Can you work these out from the model? Positions are in its coordinate system, mm. Give positions to 0.01 mm unless a question says otherwise; leave off trailing zeros. Loops run counter-clockwise (first coordinate to the right, second up) from the corner with the lowest first, then second, coordinate; pieces in that order, holes last. Notation, with made-up numbers: (-4.75, 23.25) - (12.25, 23.25) arc R27 ccw to (12.25, 53.25) - close; hole circle Ø6 at (-21, 11). An arc over 180 degrees is marked (long way). Answer in a Markdown table with one row per item.
Solid Edge part; units mm, degrees
sketch "Sketch1" plane through (0, 0, 0) normal (1, 0, 0) x (0, 1, 0)
  line L0 (0, 11) -> (17.9215, 11)
  line L1 (20, 9.8) -> (17.9215, 11)
  line L2 (20, 0) -> (20, 9.8)
  line L3 (0, 0) -> (20, 0)
  line L4 (0, 0) -> (0, 11)
revolve "RevolvedProtrusion1" add sketch "Sketch1" angle 360 about axis through (0, -25, 0) along (0, 1, 0)
chamfer "Chaflán_1" distance 0.2 angle 45 1 edges at (0, 0, 11)
hole "Agujero_1" at (0, 0, 0) direction (0, 1, 0) diameter 17 end up to next
Q1. If we mould it in two halves opening along X, with no side actions, what happens to faces 1 (the face through (9, 20, 0)), 2 (the face through (-10.74, 9.18, -2.38)), 3 (the face through (7.167, 9.86, -4.57))? For each: released by +X, released by -X, zero draft, split by the parting line, or undercut.
Checked values:
| item | result |
|---|---|
| face 1 | zero draft |
| face 2 | split by the parting line |
| face 3 | undercut |
Q2. Imagine slicing it at C-C, the plane y = 11.5. Write out the boundary of the cut face in (x, z), and give its area (3 significant figures).
Checked values:
| item | result |
|---|---|
| outline | circle Ø22 at (0, 0); hole circle Ø17 at (0, 0) |
| area | 153 mm² |
Q3. Imagine slicing it at B-B, the plane z = 0. Write out the boundary of the cut face in (x, y).
Checked values:
| item | result |
|---|---|
| outline | (-11, 0.2) - (-10.8, 0) - (-8.5, 0) - (-8.5, 20) - (-9.8, 20) - (-11, 17.92) - close; (8.5, 0) - (10.8, 0) - (11, 0.2) - (11, 17.92) - (9.8, 20) - (8.5, 20) - close |
Q4. If I drill on line 1 (X direction, y = 9.75, z = 0); line 2 (X direction, y = 7.5, z = -4), over which ranges is the centre line in solid material (lowest first)? Write a range as [from, to].
Checked values:
| item | result |
|---|---|
| line 1 | x = [-11, -8.5], [8.5, 11] |
| line 2 | x = [-10.25, -7.5], [7.5, 10.25] |
Q5. Imagine slicing it at A-A, the plane x = 0. Write out the boundary of the cut face in (y, z), and give its area (3 significant figures).
Checked values:
| item | result |
|---|---|
| outline | (0, -10.8) - (0.2, -11) - (17.92, -11) - (20, -9.8) - (20, -8.5) - (0, -8.5) - close; (0, 8.5) - (20, 8.5) - (20, 9.8) - (17.92, 11) - (0.2, 11) - (0, 10.8) - close |
| area | 97.5 mm² |
Q6. For pin 1 (1 mm diameter, centred on x = -2.5, y = 7, fed in from +Z); pin 2 (12 mm diameter, centred on y = 6, z = 7.5, fed in from +X); pin 3 (1.5 mm diameter, centred on x = -2, y = 12.5, fed in from -Z); pin 4 (10 mm diameter, centred on x = 0, z = 0, fed in from +Y), each with a flat end and sliding along its axis, tell me the tip position at first contact or that it passes through.
Checked values:
| item | result |
|---|---|
| pin 1 | stops at z = 10.82 |
| pin 2 | stops at x = 10.9 |
| pin 3 | stops at z = -10.93 |
| pin 4 | passes through |
